Part model, mm, in its own coordinate system. Round coordinates to 2 decimals unless told otherwise and drop trailing zeros. Write each loop counter-clockwise with the first axis right and the second up, starting at its lowest first coordinate (ties: lowest second). Pieces come first, ordered by that corner, then holes.
1) Saw through at B-B on z = 0. Write the cut outline in (x, y), and give its area (3 significant figures).
2) Flat gauge pins, fed straight in: pin 1 (10 mm diameter, centred on x = -2, y = 42.5, fed in from +Z); pin 2 (4 mm diameter, centred on x = -4.5, y = 52, fed in from +Z); pin 3 (0.6 mm diameter, centred on y = 21, z = 3, fed in from +X). Where does each tip first touch, or does it go through?
3) Saw through at D-D on y = 66.5. Count the separate pieces of the cut face and the enclosed holes in it, and give its area (3 significant figures).
4) Saw through at C-C on x = -6.25. Write the cut outline in (y, z).
5) Saw through at A-A on x = 0. Write the cut outline in (y, z).
6) Drill centre lines: L1, parallel to X at y = -9, z = -3.75; L2, parallel to Z at x = -7, y = -38; L3, parallel to Z at x = -8.75, y = -61.5. Where is each one in solid material? Low to high.
Autodesk Inventor part; units mm, degrees
ref_plane "YZ Plane" through (0, 0, 0) normal (1, 0, 0) x (0, 1, 0)
ref_plane "XZ Plane" through (0, 0, 0) normal (0, 1, 0) x (-1, 0, 0)
ref_plane "XY Plane" through (0, 0, 0) normal (0, 0, 1) x (1, 0, 0)
sketch "スケッチ" plane through (0, 0, 0) normal (0, 1, 0) x (-1, 0, 0)
  line L0 (8.5, -3.8) -> (8.5, -2.6)
  line L1 (4, -8.3) -> (4, -5)
  circle A0 centre (7, -7) radius 2
  line L2 (10, -2.6) -> (10, -9.5)
  line L3 (2.6, -10) -> (9.5, -10)
  line L4 (2.1, -9.5) -> (2.1, -9)
  line L5 (8.5, -2.1) -> (8.5, -4)
  line L6 (3.8, -4.8) -> (2.6, -4.8)
  line L7 (4.8, -3.8) -> (4.8, -2.6)
  arc A1 (2.1, -4.3) -> (2.6, -4.8) centre (2.6, -4.3) ccw
  arc A2 (2.6, -8.5) -> (2.1, -9) centre (2.6, -9) ccw
  arc A3 (3.8, -8.5) -> (4, -8.3) centre (3.8, -8.3) ccw
  arc A4 (4, -5) -> (3.8, -4.8) centre (3.8, -5) ccw
  arc A5 (2.1, -3.5) -> (1.6, -3) centre (1.6, -3.5) ccw
  arc A6 (2.1, -9.5) -> (2.6, -10) centre (2.6, -9.5) ccw
  arc A7 (9.5, -10) -> (10, -9.5) centre (9.5, -9.5) ccw
  arc A8 (10, -2.6) -> (9.5, -2.1) centre (9.5, -2.6) ccw
  arc A9 (9, -2.1) -> (8.5, -2.6) centre (9, -2.6) ccw
  arc A10 (8.3, -4) -> (8.5, -3.8) centre (8.3, -3.8) ccw
  arc A11 (4.8, -3.8) -> (5, -4) centre (5, -3.8) ccw
  line L8 (4.3, -2.1) -> (3.5, -2.1)
  arc A12 (4.8, -2.6) -> (4.3, -2.1) centre (4.3, -2.6) ccw
  arc A13 (3, -1.6) -> (3.5, -2.1) centre (3.5, -1.6) ccw
  line L9 (2.1, -4.3) -> (2.1, -3.5)
  line L10 (3.8, -8.5) -> (2.6, -8.5)
  line L11 (9.5, -2.1) -> (9, -2.1)
  line L12 (8.3, -4) -> (5, -4)
  circle A14 centre (0, 0) radius 1.65
  arc A15 (8.5, 2.6) -> (9, 2.1) centre (9, 2.6) ccw
  line L13 (8.5, 3.8) -> (8.5, 2.6)
  arc A16 (8.5, 3.8) -> (8.3, 4) centre (8.3, 3.8) ccw
  line L14 (8.3, 4) -> (5, 4)
  line L15 (10, 2.6) -> (10, 9.5)
  arc A17 (10, 9.5) -> (9.5, 10) centre (9.5, 9.5) ccw
  circle A18 centre (7, 7) radius 2
  line L16 (4, 8.3) -> (4, 5)
  line L17 (2.6, 10) -> (9.5, 10)
  line L18 (9.5, 2.1) -> (9, 2.1)
  arc A19 (9.5, 2.1) -> (10, 2.6) centre (9.5, 2.6) ccw
  line L19 (3.8, 8.5) -> (2.6, 8.5)
  line L20 (4.8, 3.8) -> (4.8, 2.6)
  arc A20 (4.3, 2.1) -> (4.8, 2.6) centre (4.3, 2.6) ccw
  line L21 (2.1, 8.5) -> (4, 8.5)
  arc A21 (4, 8.3) -> (3.8, 8.5) centre (3.8, 8.3) ccw
  arc A22 (2.1, 9) -> (2.6, 8.5) centre (2.6, 9) ccw
  arc A23 (2.6, 10) -> (2.1, 9.5) centre (2.6, 9.5) ccw
  line L22 (2.1, 9.5) -> (2.1, 9)
  arc A24 (1.6, 3) -> (2.1, 3.5) centre (1.6, 3.5) ccw
  line L23 (3.8, 4.8) -> (2.6, 4.8)
  arc A25 (5, 4) -> (4.8, 3.8) centre (5, 3.8) ccw
  arc A26 (3.8, 4.8) -> (4, 5) centre (3.8, 5) ccw
  line L24 (4.3, 2.1) -> (3.5, 2.1)
  arc A27 (2.6, 4.8) -> (2.1, 4.3) centre (2.6, 4.3) ccw
  line L25 (2.1, 4.3) -> (2.1, 3.5)
  arc A28 (3.5, 2.1) -> (3, 1.6) centre (3.5, 1.6) ccw
  arc A29 (-2.6, 8.5) -> (-2.1, 9) centre (-2.6, 9) ccw
  line L26 (-3.8, 8.5) -> (-2.6, 8.5)
  arc A30 (-3.8, 8.5) -> (-4, 8.3) centre (-3.8, 8.3) ccw
  line L27 (-4, 8.3) -> (-4, 5)
  line L28 (-2.6, 10) -> (-9.5, 10)
  arc A31 (-9.5, 10) -> (-10, 9.5) centre (-9.5, 9.5) ccw
  circle A32 centre (-7, 7) radius 2
  line L29 (-8.3, 4) -> (-5, 4)
  line L30 (-10, 2.6) -> (-10, 9.5)
  line L31 (-2.1, 9.5) -> (-2.1, 9)
  arc A33 (-2.1, 9.5) -> (-2.6, 10) centre (-2.6, 9.5) ccw
  line L32 (-8.5, 3.8) -> (-8.5, 2.6)
  line L33 (-3.8, 4.8) -> (-2.6, 4.8)
  arc A34 (-2.1, 4.3) -> (-2.6, 4.8) centre (-2.6, 4.3) ccw
  line L34 (-8.5, 2.1) -> (-8.5, 4)
  arc A35 (-8.3, 4) -> (-8.5, 3.8) centre (-8.3, 3.8) ccw
  arc A36 (-9, 2.1) -> (-8.5, 2.6) centre (-9, 2.6) ccw
  arc A37 (-10, 2.6) -> (-9.5, 2.1) centre (-9.5, 2.6) ccw
  line L35 (-9.5, 2.1) -> (-9, 2.1)
  arc A38 (-3, 1.6) -> (-3.5, 2.1) centre (-3.5, 1.6) ccw
  line L36 (-4.8, 3.8) -> (-4.8, 2.6)
  arc A39 (-4, 5) -> (-3.8, 4.8) centre (-3.8, 5) ccw
  arc A40 (-4.8, 3.8) -> (-5, 4) centre (-5, 3.8) ccw
  line L37 (-2.1, 4.3) -> (-2.1, 3.5)
  arc A41 (-4.8, 2.6) -> (-4.3, 2.1) centre (-4.3, 2.6) ccw
  line L38 (-4.3, 2.1) -> (-3.5, 2.1)
  arc A42 (-2.1, 3.5) -> (-1.6, 3) centre (-1.6, 3.5) ccw
  arc A43 (-8.5, -2.6) -> (-9, -2.1) centre (-9, -2.6) ccw
  line L39 (-8.5, -3.8) -> (-8.5, -2.6)
  arc A44 (-8.5, -3.8) -> (-8.3, -4) centre (-8.3, -3.8) ccw
  line L40 (-8.3, -4) -> (-5, -4)
  line L41 (-10, -2.6) -> (-10, -9.5)
  arc A45 (-10, -9.5) -> (-9.5, -10) centre (-9.5, -9.5) ccw
  circle A46 centre (-7, -7) radius 2
  line L42 (-4, -8.3) -> (-4, -5)
  line L43 (-2.6, -10) -> (-9.5, -10)
  line L44 (-9.5, -2.1) -> (-9, -2.1)
  arc A47 (-9.5, -2.1) -> (-10, -2.6) centre (-9.5, -2.6) ccw
  line L45 (-3.8, -8.5) -> (-2.6, -8.5)
  line L46 (-4.8, -3.8) -> (-4.8, -2.6)
  arc A48 (-4.3, -2.1) -> (-4.8, -2.6) centre (-4.3, -2.6) ccw
  line L47 (-2.1, -8.5) -> (-4, -8.5)
  arc A49 (-4, -8.3) -> (-3.8, -8.5) centre (-3.8, -8.3) ccw
  arc A50 (-2.1, -9) -> (-2.6, -8.5) centre (-2.6, -9) ccw
  arc A51 (-2.6, -10) -> (-2.1, -9.5) centre (-2.6, -9.5) ccw
  line L48 (-2.1, -9.5) -> (-2.1, -9)
  arc A52 (-1.6, -3) -> (-2.1, -3.5) centre (-1.6, -3.5) ccw
  line L49 (-3.8, -4.8) -> (-2.6, -4.8)
  arc A53 (-5, -4) -> (-4.8, -3.8) centre (-5, -3.8) ccw
  arc A54 (-3.8, -4.8) -> (-4, -5) centre (-3.8, -5) ccw
  line L50 (-4.3, -2.1) -> (-3.5, -2.1)
  arc A55 (-2.6, -4.8) -> (-2.1, -4.3) centre (-2.6, -4.3) ccw
  line L51 (-2.1, -4.3) -> (-2.1, -3.5)
  arc A56 (-3.5, -2.1) -> (-3, -1.6) centre (-3.5, -1.6) ccw
  line L52 (1.6, -3) -> (-1.6, -3)
  line L53 (-3, -1.6) -> (-3, 1.6)
  line L54 (-1.6, 3) -> (1.6, 3)
  line L55 (3, 1.6) -> (3, -1.6)
  point P0 (2.1, -10)
  point P1 (10, 2.1)
  point P2 (-2.1, 10)
  point P3 (-10, -2.1)
  dimension "d12" = 4
  dimension "d14" = 3.7
  dimension "d16" = 0.5
  dimension "d17" = 0.5
  dimension "d18" = 0.2
  dimension "d19" = 0.5
  dimension "d20" = 0.5
  dimension "d24" = 0.5
  dimension "d25" = 0.2
  dimension "d28" = 0.5
  dimension "d31" = 1.5
  dimension "d36" = 3.7
  dimension "d37" = 1.5
  dimension "d58" = 3.3
  dimension "d65" = 10
  dimension "d67" = 2.1
  dimension "d68" = 2.1
  dimension "d69" = 1.9
  dimension "d70" = 7
  dimension "d72" = 2.1
  dimension "d73" = 2.1
  dimension "d74" = 1.9
  dimension "d75" = 7
  dimension "d76" = 10
  dimension "d80" = 360
  dimension "d82" = 3
extrude "ボディ" add sketch "スケッチ" along normal mid plane 150
sketch "スケッチ4" plane through (0, 0, 0) normal (0, 1, 0) x (-1, 0, 0)
  line L0 (0, 0) -> (10, 0)
ref_plane "作業平面4" through (0, 0, 0) normal (0, 0, -1) x (-1, 0, 0)
sketch "スケッチ5" plane through (0, 0, 0) normal (0, 0, -1) x (-1, 0, 0)
  line L0 (-2, 0) -> (12, 0)
  line L1 (-2, 150) -> (12, 150)
sketch "スケッチ9" plane through (2.6, 0, -10) normal (0, -1, 0) x (1, 0, 0)
  circle A0 centre (4.4, 3) radius 2
  circle A1 centre (4.4, 17) radius 2
  circle A2 centre (-9.6, 17) radius 2
  circle A3 centre (-9.6, 3) radius 2
  circle A4 centre (-2.6, 10) radius 1.65
  arc A5 (-5.2, 5.2) -> (-4.7, 5.7) centre (-5.2, 5.7) ccw
  line L0 (-4.7, 5.7) -> (-4.7, 6.5)
  arc A6 (-4.2, 7) -> (-4.7, 6.5) centre (-4.2, 6.5) ccw
  line L1 (-4.2, 7) -> (-1, 7)
  arc A7 (-0.5, 6.5) -> (-1, 7) centre (-1, 6.5) ccw
  line L2 (-0.5, 6.5) -> (-0.5, 5.7)
  arc A8 (-0.5, 5.7) -> (0, 5.2) centre (0, 5.7) ccw
  line L3 (0, 5.2) -> (1.2, 5.2)
  arc A9 (1.4, 5) -> (1.2, 5.2) centre (1.2, 5) ccw
  line L4 (1.4, 5) -> (1.4, 1.7)
  arc A10 (1.2, 1.5) -> (1.4, 1.7) centre (1.2, 1.7) ccw
  line L5 (1.2, 1.5) -> (0, 1.5)
  arc A11 (0, 1.5) -> (-0.5, 1) centre (0, 1) ccw
  line L6 (-0.5, 1) -> (-0.5, 0.5)
  arc A12 (-0.5, 0.5) -> (0, 0) centre (0, 0.5) ccw
  line L7 (0, 0) -> (6.9, 0)
  arc A13 (6.9, 0) -> (7.4, 0.5) centre (6.9, 0.5) ccw
  line L8 (7.4, 0.5) -> (7.4, 7.4)
  arc A14 (7.4, 7.4) -> (6.9, 7.9) centre (6.9, 7.4) ccw
  line L9 (6.9, 7.9) -> (6.4, 7.9)
  arc A15 (6.4, 7.9) -> (5.9, 7.4) centre (6.4, 7.4) ccw
  line L10 (5.9, 7.4) -> (5.9, 6.2)
  arc A16 (5.7, 6) -> (5.9, 6.2) centre (5.7, 6.2) ccw
  line L11 (5.7, 6) -> (2.4, 6)
  arc A17 (2.2, 6.2) -> (2.4, 6) centre (2.4, 6.2) ccw
  line L12 (2.2, 6.2) -> (2.2, 7.4)
  arc A18 (2.2, 7.4) -> (1.7, 7.9) centre (1.7, 7.4) ccw
  line L13 (1.7, 7.9) -> (0.9, 7.9)
  arc A19 (0.4, 8.4) -> (0.9, 7.9) centre (0.9, 8.4) ccw
  line L14 (0.4, 8.4) -> (0.4, 11.6)
  arc A20 (0.9, 12.1) -> (0.4, 11.6) centre (0.9, 11.6) ccw
  line L15 (0.9, 12.1) -> (1.7, 12.1)
  arc A21 (1.7, 12.1) -> (2.2, 12.6) centre (1.7, 12.6) ccw
  line L16 (2.2, 12.6) -> (2.2, 13.8)
  arc A22 (2.4, 14) -> (2.2, 13.8) centre (2.4, 13.8) ccw
  line L17 (2.4, 14) -> (5.7, 14)
  arc A23 (5.9, 13.8) -> (5.7, 14) centre (5.7, 13.8) ccw
  line L18 (5.9, 13.8) -> (5.9, 12.6)
  arc A24 (5.9, 12.6) -> (6.4, 12.1) centre (6.4, 12.6) ccw
  line L19 (6.4, 12.1) -> (6.9, 12.1)
  arc A25 (6.9, 12.1) -> (7.4, 12.6) centre (6.9, 12.6) ccw
  line L20 (7.4, 12.6) -> (7.4, 19.5)
  arc A26 (7.4, 19.5) -> (6.9, 20) centre (6.9, 19.5) ccw
  line L21 (6.9, 20) -> (0, 20)
  arc A27 (0, 20) -> (-0.5, 19.5) centre (0, 19.5) ccw
  line L22 (-0.5, 19.5) -> (-0.5, 19)
  arc A28 (-0.5, 19) -> (0, 18.5) centre (0, 19) ccw
  line L23 (0, 18.5) -> (1.2, 18.5)
  arc A29 (1.4, 18.3) -> (1.2, 18.5) centre (1.2, 18.3) ccw
  line L24 (1.4, 18.3) -> (1.4, 15)
  arc A30 (1.2, 14.8) -> (1.4, 15) centre (1.2, 15) ccw
  line L25 (1.2, 14.8) -> (0, 14.8)
  arc A31 (0, 14.8) -> (-0.5, 14.3) centre (0, 14.3) ccw
  line L26 (-0.5, 14.3) -> (-0.5, 13.5)
  arc A32 (-1, 13) -> (-0.5, 13.5) centre (-1, 13.5) ccw
  line L27 (-1, 13) -> (-4.2, 13)
  arc A33 (-4.7, 13.5) -> (-4.2, 13) centre (-4.2, 13.5) ccw
  line L28 (-4.7, 13.5) -> (-4.7, 14.3)
  arc A34 (-4.7, 14.3) -> (-5.2, 14.8) centre (-5.2, 14.3) ccw
  line L29 (-5.2, 14.8) -> (-6.4, 14.8)
  arc A35 (-6.6, 15) -> (-6.4, 14.8) centre (-6.4, 15) ccw
  line L30 (-6.6, 15) -> (-6.6, 18.3)
  arc A36 (-6.4, 18.5) -> (-6.6, 18.3) centre (-6.4, 18.3) ccw
  line L31 (-6.4, 18.5) -> (-5.2, 18.5)
  arc A37 (-5.2, 18.5) -> (-4.7, 19) centre (-5.2, 19) ccw
  line L32 (-4.7, 19) -> (-4.7, 19.5)
  arc A38 (-4.7, 19.5) -> (-5.2, 20) centre (-5.2, 19.5) ccw
  line L33 (-5.2, 20) -> (-12.1, 20)
  arc A39 (-12.1, 20) -> (-12.6, 19.5) centre (-12.1, 19.5) ccw
  line L34 (-12.6, 19.5) -> (-12.6, 12.6)
  arc A40 (-12.6, 12.6) -> (-12.1, 12.1) centre (-12.1, 12.6) ccw
  line L35 (-12.1, 12.1) -> (-11.6, 12.1)
  arc A41 (-11.6, 12.1) -> (-11.1, 12.6) centre (-11.6, 12.6) ccw
  line L36 (-11.1, 12.6) -> (-11.1, 13.8)
  arc A42 (-10.9, 14) -> (-11.1, 13.8) centre (-10.9, 13.8) ccw
  line L37 (-10.9, 14) -> (-7.6, 14)
  arc A43 (-7.4, 13.8) -> (-7.6, 14) centre (-7.6, 13.8) ccw
  line L38 (-7.4, 13.8) -> (-7.4, 12.6)
  arc A44 (-7.4, 12.6) -> (-6.9, 12.1) centre (-6.9, 12.6) ccw
  line L39 (-6.9, 12.1) -> (-6.1, 12.1)
  arc A45 (-5.6, 11.6) -> (-6.1, 12.1) centre (-6.1, 11.6) ccw
  line L40 (-5.6, 11.6) -> (-5.6, 8.4)
  arc A46 (-6.1, 7.9) -> (-5.6, 8.4) centre (-6.1, 8.4) ccw
  line L41 (-6.1, 7.9) -> (-6.9, 7.9)
  arc A47 (-6.9, 7.9) -> (-7.4, 7.4) centre (-6.9, 7.4) ccw
  line L42 (-7.4, 7.4) -> (-7.4, 6.2)
  arc A48 (-7.6, 6) -> (-7.4, 6.2) centre (-7.6, 6.2) ccw
  line L43 (-7.6, 6) -> (-10.9, 6)
  arc A49 (-11.1, 6.2) -> (-10.9, 6) centre (-10.9, 6.2) ccw
  line L44 (-11.1, 6.2) -> (-11.1, 7.4)
  arc A50 (-11.1, 7.4) -> (-11.6, 7.9) centre (-11.6, 7.4) ccw
  line L45 (-11.6, 7.9) -> (-12.1, 7.9)
  arc A51 (-12.1, 7.9) -> (-12.6, 7.4) centre (-12.1, 7.4) ccw
  line L46 (-12.6, 7.4) -> (-12.6, 0.5)
  arc A52 (-12.6, 0.5) -> (-12.1, 0) centre (-12.1, 0.5) ccw
  line L47 (-12.1, 0) -> (-5.2, 0)
  arc A53 (-5.2, 0) -> (-4.7, 0.5) centre (-5.2, 0.5) ccw
  line L48 (-4.7, 0.5) -> (-4.7, 1)
  arc A54 (-4.7, 1) -> (-5.2, 1.5) centre (-5.2, 1) ccw
  line L49 (-5.2, 1.5) -> (-6.4, 1.5)
  arc A55 (-6.6, 1.7) -> (-6.4, 1.5) centre (-6.4, 1.7) ccw
  line L50 (-6.6, 1.7) -> (-6.6, 5)
  arc A56 (-6.4, 5.2) -> (-6.6, 5) centre (-6.4, 5) ccw
  line L51 (-6.4, 5.2) -> (-5.2, 5.2)
  line L52 (6.9, 20) -> (0, 20)
  line L53 (-5.2, 20) -> (0, 20)
  line L54 (7.4, 12.6) -> (7.4, 19.5)
  line L55 (7.4, 12.6) -> (7.4, 7.4)
extrude "押し出し7" add sketch "スケッチ9" along normal mid plane 150 contours A1 | A14 L9 A15 L10 A16 L11 A17 L12 A18 L13 A19 L14 A20 L15 A21 L16 A22 L17 A23 L18 A24 L19 A25 L55 | A27 L22 A28 L23 A29 L24 A30 L25 A31 L26 A32 L27 A33 L28 A34 L29 A35 L30 A36 L31 A37 L32 A38 L53
sketch "スケッチ10" plane through (-9.5, 0, 10) normal (0, -1, 0) x (1, 0, 0)
  line L0 (-0.5, -12.6) -> (-0.5, -19.5) construction
  line L1 (0, -20) -> (6.9, -20) construction
  arc A0 (-0.5, -19.5) -> (0, -20) centre (0, -19.5) ccw construction
  line L2 (-0.5, -19.5) -> (-0.5, -20) construction
  line L3 (-0.5, -20) -> (0, -20) construction
  arc A1 (0, 0) -> (-0.5, -0.5) centre (0, -0.5) ccw
  arc A2 (19.4953, -19.5681) -> (-0.0681, -0.0047) centre (-0.5, -20) ccw
  line L4 (19, 0) -> (0, 0)
  arc A3 (19.5, -0.5) -> (19, 0) centre (19, -0.5) ccw
  line L5 (19.5, -19.5) -> (19.5, -0.5)
  arc A4 (19, -20) -> (19.5, -19.5) centre (19, -19.5) ccw
  point P0 (9.5, -10)
  dimension "d101" = 20
extrude "押し出し8" cut sketch "スケッチ10" along normal through all both and the other way through all
equation "\"d99\" = Length"
equation "\"Length\" = 150"
equation "\"G_OFFSET_START\" = 0"
equation "\"G_OFFSET_END\" = 0"
equation "\"G_L\" = 150"
properties part number "r150" material "アルミニウム 6061"
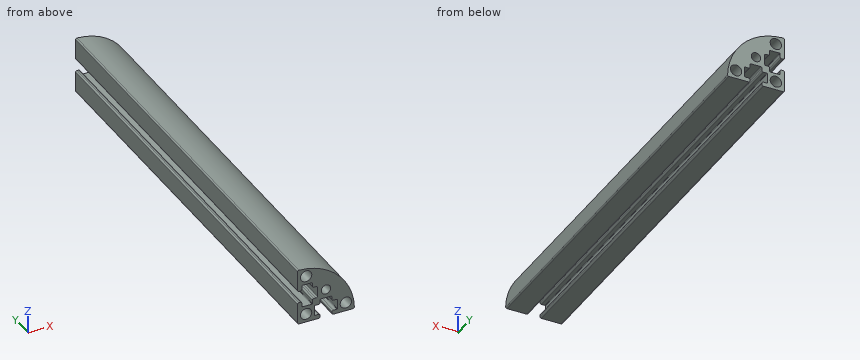
Completed:
1. outline: (-3, -75) - (-1.65, -75) - (-1.65, 75) - (-3, 75) - close; (1.65, -75) - (7.32, -75) - (7.32, 75) - (1.65, 75) - close
1. area: 1,050 mm2
2. pin 1: stops at z = 9.77
2. pin 2: stops at z = 9.69
2. pin 3: stops at x = 5.45
3. separate pieces: 1
3. enclosed holes: 4
3. area: 180 mm2
4. outline: (-75, -10) - (75, -10) - (75, -8.85) - (-75, -8.85) - close; (-75, -5.15) - (75, -5.15) - (75, -4) - (-75, -4) - close; (-75, 4) - (75, 4) - (75, 5.15) - (-75, 5.15) - close; (-75, 8.85) - (75, 8.85) - (75, 9.65) - (-75, 9.65) - close
5. outline: (-75, -3) - (75, -3) - (75, -1.65) - (-75, -1.65) - close; (-75, 1.65) - (75, 1.65) - (75, 7.32) - (-75, 7.32) - close
6. L1: x = -10 to -8.5, -4.8 to -2.1, 2.1 to 9
6. L2: z = -10 to -9, -5 to -4, 4 to 5, 9 to 9.77
6. L3: z = -10 to -7.97, -6.03 to -2.17, 2.17 to 6.03, 7.97 to 9.96
